Could you check a few things on this drawing? It's one solid part, dimensions in mm from its lowest x, y, z. A direction names the side the tool comes from. Round coordinates to 2 decimals unless told otherwise and drop trailing zeros. Write each loop counter-clockwise with the first axis right and the second up, starting at its lowest first coordinate (ties: lowest second). Pieces come first, ordered by that corner, then holes. Notation, with made-up numbers: (53.5, 38.25) - (94.5, 38.25) arc R31 ccw to (94.5, 62.25) - close; hole circle Ø3 at (80, 73.5). An arc over 180 degrees is marked (long way). Write item = value, one per line. Start each with the question number.
Item 1: If we section it at A-A (z = 32.5): Please give me the cut outline in (x, y).
Item 2: Which directions (+Z, -Z, +X, -X, +Y, -Y) give clear straight access to the entire face, cutting with the end or side of a thin tool? Please do the marked faces 1 and 2.
Item 3: If we section it at C-C (x = 20): Please give me the cut outline in (y, z), and give its area (3 significant figures).
Item 4: If we section it at B-B (x = 37.5): Please give me the cut outline in (y, z), and give its area (3 significant figures).
Item 5: If I drill on line 1 along X through (y, z) = (77.15, 32.5); line 2 along Z through (x, y) = (20, 78); line 3 along Z through (x, y) = (37.5, 76.4), over which ranges is the centre line in solid material (lowest first)? Write a range as [from, to].
Item 6: If we section it at D-D (z = 57.5): Please give me the cut outline in (x, y), and give its area (3 significant figures).
Item 7: For P1, Ø6, axis at x = 9.5, z = 8, coming from the -Y side; P2, Ø4, axis at x = 20, z = 7.5, coming from the +Y side; P3, Ø8, axis at x = 9, y = 9.5, coming from the -Z side, each with a flat end and sliding along its axis, tell me the tip position at first contact or that it passes through.
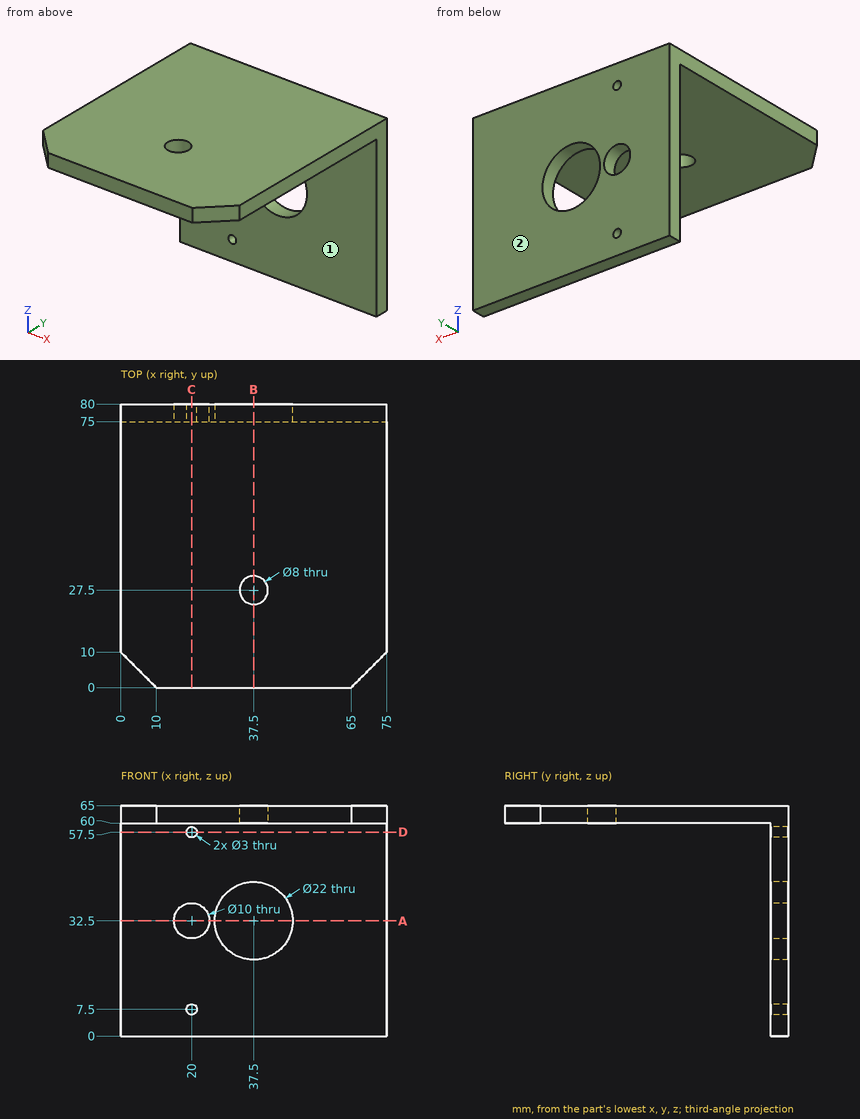
Reply:
q1.outline = (0, 75) - (15, 75) - (15, 80) - (0, 80) - close; (25, 75) - (26.5, 75) - (26.5, 80) - (25, 80) - close; (48.5, 75) - (75, 75) - (75, 80) - (48.5, 80) - close
q2.face_1 = -Z, +X, -X, -Y
q2.face_2 = +Z, -Z, +X, -X, +Y
q3.outline = (0, 60) - (75, 60) - (75, 59) - (80, 59) - (80, 65) - (0, 65) - close; (75, 0) - (80, 0) - (80, 6) - (75, 6) - close; (75, 9) - (80, 9) - (80, 27.5) - (75, 27.5) - close; (75, 37.5) - (80, 37.5) - (80, 56) - (75, 56) - close
q3.area = 620 mm2
q4.outline = (0, 60) - (23.5, 60) - (23.5, 65) - (0, 65) - close; (31.5, 60) - (75, 60) - (75, 43.5) - (80, 43.5) - (80, 65) - (31.5, 65) - close; (75, 0) - (80, 0) - (80, 21.5) - (75, 21.5) - close
q4.area = 550 mm2
q5.line_1 = [0, 15], [25, 26.5], [48.5, 75]
q5.line_2 = [0, 6], [9, 27.5], [37.5, 56], [59, 65]
q5.line_3 = [0, 21.5], [43.5, 65]
q6.outline = (0, 75) - (18.5, 75) - (18.5, 80) - (0, 80) - close; (21.5, 75) - (75, 75) - (75, 80) - (21.5, 80) - close
q6.area = 360 mm2
q7.P1 = 75
q7.P2 = 80
q7.P3 = 60
